For this review, take the finished solid that the model builds, in its own axes (mm). A direction names the side the tool comes from. Round coordinates to 2 decimals unless told otherwise and drop trailing zeros. Order: outer loops, then holes, each group sorted by start corner. A loop starts at its lowest first (then second) coordinate and runs counter-clockwise, first axis right, second up. Notation, with made-up numbers: (-39, -39.75) - (-8, -39.75) arc R19 ccw to (-8, -4.75) - close; hole circle Ø5 at (42, 51.5). An arc over 180 degrees is marked (long way). One line per item, written item: value.
```python
from build123d import *

# Parameters (mm, degrees)
SKETCH1_W           = 41.5
SKETCH1_H           = 22
BASE_DEPTH          = 13.5
FILLET1_R           = 2
SKETCH2_R           = 1.1
SCREWHOLE_DEPTH     = 13.5
SKETCH3_R           = 2.5
SPINAXEL_DEPTH      = 9
SKETCH4_R           = 1.8
FITTINGKNOB_DEPTH   = 1.8
BOSS_EXTRUDE4_DEPTH = 36
EXTRUDE_THIN1_DEPTH = 2
SKETCH7_W           = 3.5
SKETCH7_H           = 8
BOSS_EXTRUDE5_DEPTH = 8
FILLET2_RADIUS      = 1.75
FILLET2_LENGTH      = 8


# Read off the part's stored shape, not the designer's step: Extrude-Thin1
with BuildPart() as part:
    # Sketch1 → Base (new body)
    with BuildSketch(Plane(origin=(0, 0, 0), x_dir=(1, 0, 0), z_dir=(0, 1, 0))):
        Rectangle(SKETCH1_W, SKETCH1_H)
    extrude(amount=BASE_DEPTH)

    # Fillet1
    fillet1_edges = [part.edges().sort_by_distance(p)[0] for p in [
        (20.75, 6.75, 11),
        (-20.75, 6.75, 11),
        (-20.75, 6.75, -11),
        (20.75, 6.75, -11),
    ]]
    fillet(fillet1_edges, radius=FILLET1_R)

    # Sketch2 → ScrewHole (cut)
    with BuildSketch(Plane(origin=(0, 13.5, 0), x_dir=(1, 0, 0), z_dir=(0, 1, 0))):
        with Locations(Location((-18.75, 9, 0), (0, 0, 270))):
            Circle(SKETCH2_R)
        with Locations(Location((-18.75, -9, 0), (0, 0, 270))):
            Circle(SKETCH2_R)
    extrude(amount=-SCREWHOLE_DEPTH, mode=Mode.SUBTRACT)

    # Sketch3 → SpinAxel (add)
    with BuildSketch(Plane(origin=(0, 13.5, 0), x_dir=(1, 0, 0), z_dir=(0, 1, 0))):
        with Locations(Location((-9.75, 0, 0), (0, 0, 270))):
            Circle(SKETCH3_R)
    extrude(amount=SPINAXEL_DEPTH)

    # Sketch4 → FittingKnob (add)
    with BuildSketch(Plane(origin=(0, 13.5, 0), x_dir=(1, 0, 0), z_dir=(0, 1, 0))):
        with Locations(Location((1.25, 0, 0), (0, 0, 270))):
            Circle(SKETCH4_R)
    extrude(amount=FITTINGKNOB_DEPTH)

    # Sketch5 → Boss-Extrude4 (add)
    with BuildSketch(Plane(origin=(0, 0, 0), x_dir=(-1, 0, 0), z_dir=(0, -1, 0))):
        with BuildLine():
            Line((-3.75, -6.982120022), (-3.75, 6.982120022))
            ThreePointArc((-3.75, 6.982120022), (-12.25, 11), (-20.75, 6.982120022))
            Line((-20.75, 6.982120022), (-20.75, -6.982120022))
            ThreePointArc((-20.75, -6.982120022), (-12.25, -11), (-3.75, -6.982120022))
        make_face()
    extrude(amount=BOSS_EXTRUDE4_DEPTH)

    # Extrude-Thin1 outline → Extrude-Thin1 (add)
    with BuildSketch(Plane(origin=(0, -26, 0), x_dir=(-1, 0, 0), z_dir=(0, -1, 0))):
        with BuildLine():
            ThreePointArc((-3.75, -6.982120022), (-10.984143444, -10.926921212), (-18.928571429, -8.740519646))
            Line((-18.928571429, -8.740519646), (-20.75, -11.124297731))
            ThreePointArc((-20.75, -11.124297731), (-10.882966454, -13.933097979), (-1.75, -9.260129589))
            Line((-1.75, -9.260129589), (9.25, -9.260129589))
            Line((9.25, -9.260129589), (9.25, 9.260129589))
            Line((9.25, 9.260129589), (-1.75, 9.260129589))
            ThreePointArc((-1.75, 9.260129589), (-10.882966454, 13.933097979), (-20.75, 11.124297731))
            Line((-20.75, 11.124297731), (-18.928571429, 8.740519646))
            ThreePointArc((-18.928571429, 8.740519646), (-10.984143444, 10.926921212), (-3.75, 6.982120022))
            Line((-3.75, 6.982120022), (-3.75, -6.982120022))
        make_face()
    extrude(amount=EXTRUDE_THIN1_DEPTH)

    # Sketch7 → Boss-Extrude5 (add)
    with BuildSketch(Plane(origin=(20.75, 0, 0), x_dir=(0, 0, -1), z_dir=(1, 0, 0))):
        with Locations((0, -4)):
            Rectangle(SKETCH7_W, SKETCH7_H)
    extrude(amount=BOSS_EXTRUDE5_DEPTH)

    # Fillet2: full round fillet: the end face becomes a half cylinder, R = half its width
    fillet2_face = Plane((28.75, -4, 0), x_dir=(0, 1, 0), z_dir=(1, 0, 0))  # on the end face: x along it, z out of the body
    fillet2_slab = fillet2_face.offset(-FILLET2_RADIUS / 2) * Box(FILLET2_LENGTH, 2 * FILLET2_RADIUS, FILLET2_RADIUS, mode=Mode.PRIVATE)  # the body's end, R deep
    fillet2_round = Plane((27, -4, 0), x_dir=(1, 0, 0), z_dir=(0, 1, 0)) * Cylinder(FILLET2_RADIUS, FILLET2_LENGTH, mode=Mode.PRIVATE)  # its axis R under the face
    add(fillet2_slab - fillet2_round, mode=Mode.SUBTRACT)


solid = part.part
```
Item 1: For P1, Ø6, axis at x = -2, y = -28, coming from the +Z side; P2, Ø2, axis at y = -26.5, z = 1, coming from the -X side; P3, Ø1.8, axis at x = 23, z = 0, coming from the -Y side, all flat-tipped, find the tip position at first contact; note any pin that passes through.
Returned:
P1: z = 9.26
P2: x = -9.25
P3: y = -8
Item 2: Take a section at B-B (z = 0). Write out the cut boundary in (x, y).
Returned:
outline: (-20.75, 0) - (3.75, 0) - (3.75, -26) - (-9.25, -26) - (-9.25, -28) - (3.75, -28) - (3.75, -36) - (20.75, -36) - (20.75, -8) - (28.75, -8) - (28.75, 0) - (20.75, 0) - (20.75, 13.5) - (3.05, 13.5) - (3.05, 15.3) - (-0.55, 15.3) - (-0.55, 13.5) - (-7.25, 13.5) - (-7.25, 22.5) - (-12.25, 22.5) - (-12.25, 13.5) - (-20.75, 13.5) - close
Item 3: Wall thickness on line 1 (Y direction, x = 4.5, z = -8.75); line 2 (X direction, y = 6.5, z = -9); line 3 (Z direction, x = -18, y = 3): over which ranges is each line inside the solid? List them lowest first.
Returned:
line 1: -28 to -26, 0 to 13.5
line 2: -20.75 to -19.85, -17.65 to 20.75
line 3: -11 to -9.8, -8.2 to 8.2, 9.8 to 11
Item 4: Take a section at D-D (y = -6). Write out the cut boundary in (x, z).
Returned:
outline: (3.75, -6.98) arc R11 ccw to (20.75, -6.98) - (20.75, -1.75) - (27, -1.75) arc R1.75 ccw to (27, 1.75) - (20.75, 1.75) - (20.75, 6.98) arc R11 ccw to (3.75, 6.98) - close
Item 5: The part is to be moulded in two halves that separate along Y. For faces 5 (the flat face through (1, 15.3, 0)), 6 (the flat face through (3.75, -13, 0)), 7 (the cylindrical face through (-20.18, 6.84, 10.4)), say which applies: +Y half, -Y half, draft (parallel to the pull), parting line (faces both ways), or undercut.
Returned:
face 5: +Y half
face 6: undercut
face 7: draft
Item 6: Machinability: for faces 1 (the flat face through (24, -4, 1.75)), 2 (the flat face through (0, 7, -11)), 3 (the cylindrical face through (20.18, 6.84, -10.4)), 4 (the flat face through (-9.25, -27, 0)), which of the approach directions +Z, -Z, +X, -X, +Y, -Y give a long, thin tool a straight path to every point of the face, cutting with its end or side? Answer none if there is none.
Returned:
face 1: +Z, +X, +Y, -Y
face 2: -Z, +X, -X, +Y
face 3: -Z, +X, +Y
face 4: +Z, -Z, -X, -Y
Item 7: Take a section at A-A (y = 10.5). Write out the cut boundary in (x, z), plus the area to 3 significant figures.
Returned:
outline: (-20.75, -9) arc R2 ccw to (-18.75, -11) - (18.75, -11) arc R2 ccw to (20.75, -9) - (20.75, 9) arc R2 ccw to (18.75, 11) - (-18.75, 11) arc R2 ccw to (-20.75, 9) - close; hole circle Ø2.2 at (-18.75, -9); hole circle Ø2.2 at (-18.75, 9)
area: 902 mm^2
Item 8: Take a section at C-C (x = 15). Write out the cut boundary in (y, z), plus the area to 3 significant figures.
Returned:
outline: (-36, -10.65) - (-28, -10.65) - (-28, -13.73) - (-26, -13.73) - (-26, -10.65) - (0, -10.65) - (0, -11) - (13.5, -11) - (13.5, 11) - (0, 11) - (0, 10.65) - (-26, 10.65) - (-26, 13.73) - (-28, 13.73) - (-28, 10.65) - (-36, 10.65) - close
area: 1,080 mm^2
